Autodesk Inventor part; units mm, degrees
ref_plane "Work Plane1" through (-3.75, 20, 0) normal (1, 0, 0) x (0, 1, 0)
ref_plane "XZ Plane" through (0, 0, 0) normal (0, 1, 0) x (-1, 0, 0)
ref_plane "XY Plane" through (0, 0, 0) normal (0, 0, 1) x (1, 0, 0)
sketch "Sketch1" plane through (0, 0, 0) normal (0, 1, 0) x (-1, 0, 0)
  circle A0 centre (0, 0) radius 3.75
  circle A1 centre (0, 0) radius 1.5
  dimension "d0" = 7.5
  dimension "d1" = 3
extrude "Extrusion1" add sketch "Sketch1" along normal blind 4
sketch "Sketch2" plane through (0, 4, 0) normal (0, 1, 0) x (1, 0, 0)
  circle A0 centre (0, 0) radius 3.75
  circle A1 centre (0, 0) radius 3.75
  line L0 (0, 0) -> (0, 7)
  circle A2 centre (0, 7) radius 2
  line L1 (-3.6309, 0.9375) -> (-1.9365, 7.5)
  line L2 (1.9365, 7.5) -> (3.6309, 0.9375)
  circle A3 centre (0, 0) radius 1.5
  line L3 (0, 0) -> (0, -10)
  circle A4 centre (0, -10) radius 0.8
  circle A5 centre (0, -10) radius 2
  line L4 (-1.9691, -10.35) -> (-3.6921, -0.6563)
  line L5 (3.6921, -0.6562) -> (1.9691, -10.35)
  dimension "d4" = 7
  dimension "d5" = 4
  dimension "d7" = 10
  dimension "d8" = 1.6
  dimension "d9" = 4
extrude "Extrusion2" add sketch "Sketch2" along normal blind 1 contours A0 L3 A3 L0 | A0 L0 A2 L2 | L5 A5 L3 A0 | L0 A3 L3 A0 | A0 L1 A2 L0 | A2 | L3 A5 L4 A0 | A5
extrude "Extrusion3" add sketch "Sketch2" along normal blind 16 contours A2
sketch "Sketch3" plane through (0, 20, -7) normal (0, 1, 0) x (1, 0, 0)
  arc A0 (-3.6921, -7.6563) -> (3.6921, -7.6562) centre (0, -7) ccw
  arc A1 (3.6309, -6.0625) -> (-3.6309, -6.0625) centre (0, -7) ccw
  arc A2 (-3.6309, -6.0625) -> (-3.6921, -7.6563) centre (0, -7) ccw
  arc A3 (3.6921, -7.6562) -> (3.6309, -6.0625) centre (0, -7) ccw
  circle A4 centre (0, -7) radius 1.5
  line L0 (-1.9365, 0.5) -> (-3.6309, -6.0625)
  line L1 (3.6309, -6.0625) -> (1.9365, 0.5)
  circle A5 centre (0, 0) radius 2
extrude "Extrusion4" add sketch "Sketch3" along normal blind 1
extrude "Extrusion5" add sketch "Sketch3" along normal blind 5
ref_plane "Work Plane1" through (-3.75, 20, 0) normal (1, 0, 0) x (0, 1, 0)
sketch "Sketch5" plane through (-3.75, 20, 0) normal (1, 0, 0) x (0, 1, 0)
  line L0 (5, 1.5) -> (5, -1.5)
  line L1 (0, -1.5) -> (0, 1.5)
  line L2 (-15, 1.5) -> (-15, -1.5)
  line L3 (-20, -1.5) -> (-20, 1.5)
  line L4 (0, 0) -> (5, 0)
  line L5 (-15, 0) -> (-20, 0)
  circle A0 centre (-17.5, 0) radius 1.5
  circle A1 centre (2.5, 0) radius 1.5
  dimension "d19" = 3
  dimension "d20" = 3
  dimension "d27" = 20
extrude "Extrusion6" cut sketch "Sketch5" along normal up to surface
thread "Thread1"
thread "Thread2"
properties part number "steeringYoke3mmShaft" material "Brass, Soft Yellow"
Build history of the part. All positions in model axes, mm. A direction names the side the tool comes from. Round coordinates to 2 decimals unless told otherwise and drop trailing zeros. Loops run counter-clockwise (first coordinate to the right, second up) from the corner with the lowest first, then second, coordinate; pieces in that order, holes last. Notation, with made-up numbers: (58.5, 8) -> (92.5, 8) arc R28 cw to (92.5, 41) -> close; hole circle Ø7 at (-24.75, 84). An arc over 180 degrees is marked (long way). Answer in a Markdown table with one row per item.
Item 1: Saw through at A-A (x = -2.5). Write the cut outline in (y, z), and give its area (3 significant figures).
Answers below:
| item | result |
|---|---|
| outline | (0, -2.8) -> (4, -2.8) -> (4, -5.32) -> (5, -5.32) -> (5, 7.36) -> (4, 7.36) -> (4, 2.8) -> (0, 2.8) -> close; (20, -5.32) -> (25, -5.32) -> (25, 2.8) -> (20, 2.8) -> close; hole circle Ø3 at (2.5, 0); hole circle Ø3 at (22.5, 0) |
| area | 61.5 mm² |
Item 2: Saw through at D-D (y = 22.5). Write the cut outline in (x, z).
Answers below:
| item | result |
|---|---|
| outline | (-3.49, -1.5) -> (-1.94, -7.5) arc R2 ccw to (1.94, -7.5) -> (3.63, -0.94) arc R3.75 ccw to (3.69, 0.66) arc R3.75 ccw to (-3.44, 1.5) -> (0, 1.5) arc R1.5 cw to (0, -1.5) -> close |
Item 3: Pin check, flat tips, straight feed: pin 1 (4 mm diameter, centred on x = -1.5, y = 6.5, fed in from +Z); pin 2 (5 mm diameter, centred on y = 5.5, z = -6.5, fed in from -X); pin 3 (8 mm diameter, centred on y = 4.5, z = 4.5, fed in from -X). Stop position of each tip, or through.
Answers below:
| item | result |
|---|---|
| pin 1 | stops at z = 11.99 |
| pin 2 | stops at x = -2.83 |
| pin 3 | stops at x = -3.72 |
Item 4: Saw through at B-B (z = 2.5). Write the cut outline in (x, y).
Answers below:
| item | result |
|---|---|
| outline | (-3.36, 4) -> (-2.8, 4) -> (-2.8, 0) -> (2.8, 0) -> (2.8, 4) -> (3.36, 4) -> (3.36, 5) -> (-3.36, 5) -> close; (-2.8, 20) -> (2.8, 20) -> (2.8, 25) -> (-2.8, 25) -> close |
Item 5: Mould opens along Z. For faces 1 (the cylindrical face through (-2.318, 23.306, -1.265)), 2 (the cylindrical face through (1.43, 22.46, 0.45)), 3 (the flat face through (-2.82, 4.49, 5.57)), 4 (the cylindrical face through (3.747, 22.465, -0.155)) say: +Z half, -Z half, draft (parallel to the pull), parting line (faces both ways), or undercut.
Answers below:
| item | result |
|---|---|
| face 1 | undercut |
| face 2 | undercut |
| face 3 | +Z half |
| face 4 | parting line |
Item 6: Drill centre lines: L1, parallel to Y at x = -0.25, z = -2.75; L2, parallel to X at y = 22.85, z = 0; L3, parallel to X at y = 4.3, z = 10. Where is each one in solid material? Low to high. Write a range as [from, to].
Answers below:
| item | result |
|---|---|
| L1 | y = [0, 5], [20, 25] |
| L2 | x = [1.5, 3.75] |
| L3 | x = [-2.03, -0.8], [0.8, 2.03] |
Item 7: Which spindle directions (+Z, -Z, +X, -X, +Y, -Y) get a long thin tool onto all of the face, cutting with end or side? Do faces 5 (the cylindrical face through (-2.318, 3.306, -1.265)), 6 (the cylindrical face through (0, 14, -9)), 7 (the cylindrical face through (3.717, 1.909, -0.498)), 8 (the cylindrical face through (-3.748, 20.508, -0.133)). Say none if no direction does.
Answers below:
| item | result |
|---|---|
| face 5 | -X |
| face 6 | none |
| face 7 | -Y |
| face 8 | -X, +Y, -Y |
